```python
from build123d import *

# Parameters (mm, degrees)
MEMBER_1_DEPTH         = 2932
HOLE_WIZARD_M4_1_D     = 3.3
HOLE_WIZARD_M4_1_DEPTH = 10.1
HOLE_WIZARD_M4_1_TIP   = 0.991420021
HOLE_WIZARD_M4_2_D     = 3.3
HOLE_WIZARD_M4_2_DEPTH = 10.1
HOLE_WIZARD_M4_2_TIP   = 0.991420021


with BuildPart() as part:
    # Sketch1 → Member 1 (new body)
    with BuildSketch(Plane.YZ):
        with BuildLine():
            Line((-9.8, -15), (9.8, -15))
            ThreePointArc((9.8, -15), (13.476955262, -13.476955262), (15, -9.8))
            Line((15, -9.8), (15, 9.8))
            ThreePointArc((15, 9.8), (13.476955262, 13.476955262), (9.8, 15))
            Line((9.8, 15), (-9.8, 15))
            ThreePointArc((-9.8, 15), (-13.476955262, 13.476955262), (-15, 9.8))
            Line((-15, 9.8), (-15, -9.8))
            ThreePointArc((-15, -9.8), (-13.476955262, -13.476955262), (-9.8, -15))
        make_face()
        with BuildLine():
            Line((-9.8, -12.4), (9.8, -12.4))
            ThreePointArc((9.8, -12.4), (11.638477631, -11.638477631), (12.4, -9.8))
            Line((12.4, -9.8), (12.4, 9.8))
            ThreePointArc((12.4, 9.8), (11.638477631, 11.638477631), (9.8, 12.4))
            Line((9.8, 12.4), (-9.8, 12.4))
            ThreePointArc((-9.8, 12.4), (-11.638477631, 11.638477631), (-12.4, 9.8))
            Line((-12.4, 9.8), (-12.4, -9.8))
            ThreePointArc((-12.4, -9.8), (-11.638477631, -11.638477631), (-9.8, -12.4))
        make_face(mode=Mode.SUBTRACT)
    extrude(amount=MEMBER_1_DEPTH)

    # M4 螺纹孔1
    with Locations(Plane(origin=(0, -15, 0), x_dir=(-1, 0, 0), z_dir=(0, -1, 0))):
        with Locations((-20.95, 0), (-50.95, 0), (-2881.05, 0), (-2911.05, 0)):
            Hole(HOLE_WIZARD_M4_1_D / 2, depth=HOLE_WIZARD_M4_1_DEPTH)
            with Locations((0, 0, -(HOLE_WIZARD_M4_1_DEPTH + HOLE_WIZARD_M4_1_TIP / 2))):  # 118° drill point
                Cone(0, HOLE_WIZARD_M4_1_D / 2, HOLE_WIZARD_M4_1_TIP, mode=Mode.SUBTRACT)

    # M4 螺纹孔2
    with Locations(Plane.XY.offset(15)):
        with Locations((1139.95, 0), (1239.95, 0), (1339.95, 0), (1592.05, 0), (1692.05, 0), (1792.05, 0)):
            Hole(HOLE_WIZARD_M4_2_D / 2, depth=HOLE_WIZARD_M4_2_DEPTH)
            with Locations((0, 0, -(HOLE_WIZARD_M4_2_DEPTH + HOLE_WIZARD_M4_2_TIP / 2))):  # 118° drill point
                Cone(0, HOLE_WIZARD_M4_2_D / 2, HOLE_WIZARD_M4_2_TIP, mode=Mode.SUBTRACT)


solid = part.part
```
Check sheet for the modelled part. Datum: model origin and axes. Units: mm. Round coordinates to 2 decimals unless told otherwise and drop trailing zeros. Order: outer loops, then holes, each group sorted by start corner. A loop starts at its lowest first (then second) coordinate and runs counter-clockwise, first axis right, second up.
1) Section check A-A (x = 2580.5). Record the boundary of the cut face in (y, z), and give its area (3 significant figures).
2) Go/stop test with flat-tipped pins: pin 1 Ø12 at (y, z) = (-12, 0.5) entering from +X; pin 2 Ø2 at (x, y) = (1339.95, 0) entering from +Z; pin 3 Ø2.5 at (x, z) = (2911.05, 0) entering from -Y; pin 4 Ø1.5 at (y, z) = (11, -7) entering from -X. Record where each tip stops, or that it passes through.
3) Scan lines: line 1 (Y direction, x = 1767, z = 7.5); line 2 (Y direction, x = 2642, z = 10.5). Record each from-to range of solid material in increasing order.
Result:
1. outline: (-15, -9.8) arc R5.2 ccw to (-9.8, -15) - (9.8, -15) arc R5.2 ccw to (15, -9.8) - (15, 9.8) arc R5.2 ccw to (9.8, 15) - (-9.8, 15) arc R5.2 ccw to (-15, 9.8) - close; hole (-12.4, -9.8) arc R2.6 ccw to (-9.8, -12.4) - (9.8, -12.4) arc R2.6 ccw to (12.4, -9.8) - (12.4, 9.8) arc R2.6 ccw to (9.8, 12.4) - (-9.8, 12.4) arc R2.6 ccw to (-12.4, 9.8) - close
1. area: 268 mm2
2. pin 1: stops at x = 2932
2. pin 2: stops at z = -12.4
2. pin 3: stops at y = 12.4
2. pin 4: passes through
3. line 1: y = -15 to -12.4, 12.4 to 15
3. line 2: y = -14.95 to -12.3, 12.3 to 14.95
